The model under review builds one solid part; all positions refer to its coordinate system, in mm. Give positions to 0.01 mm unless a question says otherwise; leave off trailing zeros. Order: outer loops, then holes, each group sorted by start corner. A loop starts at its lowest first (then second) coordinate and runs counter-clockwise, first axis right, second up. Notation, with made-up numbers: (8, 2) - (24, 2) arc R28 cw to (24, 40) - close; hole circle Ø5 at (-9.5, -14). An arc over 180 degrees is marked (long way). Use CSV: the item, a comma, the result in double quotes. Start each with the question number.
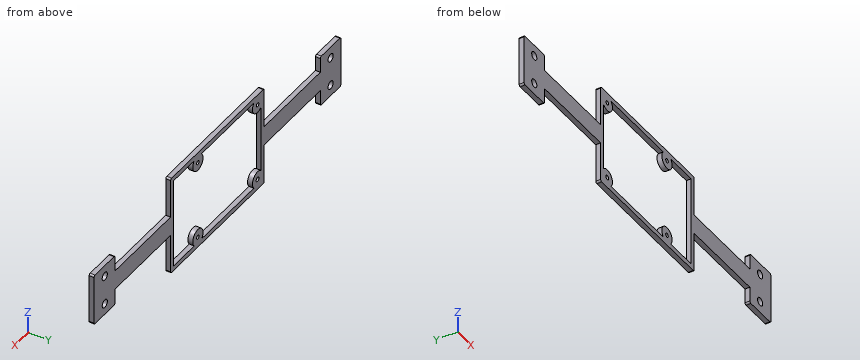
```python
from build123d import *

# Parameters (mm, degrees)
SKETCH1_W           = 91
SKETCH1_H           = 62
BOSS_EXTRUDE3_DEPTH = 3
SKETCH2_W           = 85
SKETCH2_H           = 56
CUT_EXTRUDE1_DEPTH  = 3
SKETCH3_R           = 5
SKETCH3_R_2         = 1.25
SKETCH3_R_3         = 1.35
BOSS_EXTRUDE4_DEPTH = 3
SKETCH4_W           = 12
SKETCH4_H           = 3
BOSS_EXTRUDE5_DEPTH = 54.5
SKETCH5_W           = 20
SKETCH5_H           = 32
SKETCH5_R           = 2.5
BOSS_EXTRUDE6_DEPTH = 3
SKETCH6_W           = 12
SKETCH6_H           = 3
BOSS_EXTRUDE7_DEPTH = 54.5
SKETCH7_R           = 5
SKETCH7_R_2         = 1.25
BOSS_EXTRUDE8_DEPTH = 3
SKETCH8_W           = 20.5
SKETCH8_H           = 32
SKETCH8_R           = 2.5
BOSS_EXTRUDE9_DEPTH = 3
FILLET1_R           = 1


with BuildPart() as part:
    # Sketch1 → Boss-Extrude3 (new body)
    with BuildSketch(Plane(origin=(0, 0, 0), x_dir=(1, 0, 0), z_dir=(0, 1, 0))):
        with Locations((45.5, 31)):
            Rectangle(SKETCH1_W, SKETCH1_H)
    extrude(amount=BOSS_EXTRUDE3_DEPTH)

    # Sketch2 → Cut-Extrude1 (cut)
    with BuildSketch(Plane(origin=(0, 3, 0), x_dir=(1, 0, 0), z_dir=(0, 1, 0))):
        with Locations((45.5, 31)):
            Rectangle(SKETCH2_W, SKETCH2_H)
    extrude(amount=-CUT_EXTRUDE1_DEPTH, mode=Mode.SUBTRACT)

    # Sketch3 → Boss-Extrude4 (add)
    # profile 1 of 2: a face of its own
    with BuildSketch(Plane(origin=(0, 3, 0), x_dir=(1, 0, 0), z_dir=(0, 1, 0))):
        with Locations((6.5, 6.5)):
            Circle(SKETCH3_R)
        with Locations(Location((6.5, 6.5, 0), (0, 0, 270))):
            Circle(SKETCH3_R_2, mode=Mode.SUBTRACT)
    # profile 2 of 2: a face of its own
    with BuildSketch(Plane(origin=(0, 3, 0), x_dir=(1, 0, 0), z_dir=(0, 1, 0))):
        with Locations((6.5, 55.5)):
            Circle(SKETCH3_R)
        with Locations(Location((6.5, 55.5, 0), (0, 0, 270))):
            Circle(SKETCH3_R_3, mode=Mode.SUBTRACT)
    extrude(amount=-BOSS_EXTRUDE4_DEPTH)

    # Sketch4 → Boss-Extrude5 (add)
    with BuildSketch(Plane.ZY):
        with Locations((-31, 1.5)):
            Rectangle(SKETCH4_W, SKETCH4_H)
    extrude(amount=BOSS_EXTRUDE5_DEPTH)

    # Sketch5 → Boss-Extrude6 (add)
    with BuildSketch(Plane(origin=(0, 3, 0), x_dir=(1, 0, 0), z_dir=(0, 1, 0))):
        with Locations((-64.5, 31)):
            Rectangle(SKETCH5_W, SKETCH5_H)
        with Locations(Location((-64.5, 40, 0), (0, 0, 270))):
            Circle(SKETCH5_R, mode=Mode.SUBTRACT)
        with Locations(Location((-64.5, 22, 0), (0, 0, 270))):
            Circle(SKETCH5_R, mode=Mode.SUBTRACT)
    extrude(amount=-BOSS_EXTRUDE6_DEPTH)

    # Sketch6 → Boss-Extrude7 (add)
    with BuildSketch(Plane(origin=(91, 0, 0), x_dir=(0, 0, -1), z_dir=(1, 0, 0))):
        with Locations((31, 1.5)):
            Rectangle(SKETCH6_W, SKETCH6_H)
    extrude(amount=BOSS_EXTRUDE7_DEPTH)

    # Sketch7 → Boss-Extrude8 (add)
    # profile 1 of 2: a face of its own
    with BuildSketch(Plane(origin=(0, 3, 0), x_dir=(1, 0, 0), z_dir=(0, 1, 0))):
        with Locations((64.5, 55.5)):
            Circle(SKETCH7_R)
        with Locations(Location((64.5, 55.5, 0), (0, 0, 270))):
            Circle(SKETCH7_R_2, mode=Mode.SUBTRACT)
    # profile 2 of 2: a face of its own
    with BuildSketch(Plane(origin=(0, 3, 0), x_dir=(1, 0, 0), z_dir=(0, 1, 0))):
        with Locations((64.5, 6.5)):
            Circle(SKETCH7_R)
        with Locations(Location((64.5, 6.5, 0), (0, 0, 270))):
            Circle(SKETCH7_R_2, mode=Mode.SUBTRACT)
    extrude(amount=-BOSS_EXTRUDE8_DEPTH)

    # Sketch8 → Boss-Extrude9 (add)
    with BuildSketch(Plane(origin=(0, 3, 0), x_dir=(1, 0, 0), z_dir=(0, 1, 0))):
        with Locations((155.25, 31)):
            Rectangle(SKETCH8_W, SKETCH8_H)
        with Locations(Location((155, 40, 0), (0, 0, 270))):
            Circle(SKETCH8_R, mode=Mode.SUBTRACT)
        with Locations(Location((155, 22, 0), (0, 0, 270))):
            Circle(SKETCH8_R, mode=Mode.SUBTRACT)
    extrude(amount=-BOSS_EXTRUDE9_DEPTH)

    # Fillet1
    fillet1_edges = [part.edges().sort_by_distance(p)[0] for p in [
        (145, 1.5, -15),
        (145, 1.5, -47),
        (165.5, 1.5, -47),
        (165.5, 1.5, -15),
        (-54.5, 1.5, -47),
        (-54.5, 1.5, -15),
        (-74.5, 1.5, -15),
        (-74.5, 1.5, -47),
        (0, 1.5, -62),
        (91, 1.5, -62),
        (91, 1.5, 0),
        (0, 1.5, 0),
    ]]
    fillet(fillet1_edges, radius=FILLET1_R)


solid = part.part
```
1. Consider section D-D (x = 118.5). Give the boundary of the cut face in (y, z).
2. Consider section C-C (y = 1.75). State how many separate pieces and enclosed holes the cut face has, and give its area (3 significant figures).
3. To check wall thickness, follow L1, parallel to X at y = 2.25, z = -40; L2, parallel to X at y = 0.9, z = -55.5; L3, parallel to X at y = 1.55, z = -5. State the ranges of each line that lie inside material, in increasing order. Write a range as [from, to].
4. Clearance check with flat-ended pins moving along their axes: pin 1 (1.5 mm diameter, centred on x = -25, z = -38.5, fed in from -Y); pin 2 (1.5 mm diameter, centred on y = 2, z = -55, fed in from -X); pin 3 (1.5 mm diameter, centred on y = 1.5, z = -49.5, fed in from +X). State where each tip first meets the part, or that it passes through.
5. Consider section B-B (x = -64.5). Give the boundary of the cut face in (y, z), and give its area (3 significant figures).
6. Consider section A-A (z = -40). Give the boundary of the cut face in (x, y).
Answers follow:
1,outline,"(0, -37) - (3, -37) - (3, -25) - (0, -25) - close"
2,separate pieces,"1"
2,enclosed holes,"9"
2,area,"3,650 mm^2"
3,L1,"x = [-74.5, -67], [-62, -54.5], [0, 3], [88, 91], [145, 152.5], [157.5, 165.5]"
3,L2,"x = [0, 5.15], [7.85, 11.5], [59.5, 63.25], [65.75, 69.5], [88, 91]"
3,L3,"x = [0, 11.27], [59.73, 69.27], [88, 91]"
4,pin 1,"passes through"
4,pin 2,"stops at x = 0"
4,pin 3,"stops at x = 91"
5,outline,"(0, -47) - (3, -47) - (3, -42.5) - (0, -42.5) - close; (0, -37.5) - (3, -37.5) - (3, -24.5) - (0, -24.5) - close; (0, -19.5) - (3, -19.5) - (3, -15) - (0, -15) - close"
5,area,"66.0 mm^2"
6,outline,"(-74.5, 0) - (-67, 0) - (-67, 3) - (-74.5, 3) - close; (-62, 0) - (-54.5, 0) - (-54.5, 3) - (-62, 3) - close; (0, 0) - (3, 0) - (3, 3) - (0, 3) - close; (88, 0) - (91, 0) - (91, 3) - (88, 3) - close; (145, 0) - (152.5, 0) - (152.5, 3) - (145, 3) - close; (157.5, 0) - (165.5, 0) - (165.5, 3) - (157.5, 3) - close"
